Check sheet for the modelled part. Datum: model origin and axes. Units: mm. Face numbers are marked on the shaded views. Coordinates: 2 decimals unless noted, no trailing zeros. Order: outer loops, then holes, each group sorted by start corner. A loop starts at its lowest first (then second) coordinate and runs counter-clockwise, first axis right, second up. Notation, with made-up numbers: M 67.25,-1.5 L 104.25,-1.5 A25 ccw 104.25,18.5 Z; hole C 85.25,-40 d9. An arc over 180 degrees is marked long. Answer in a Markdown table with one row per item. Add a question column.
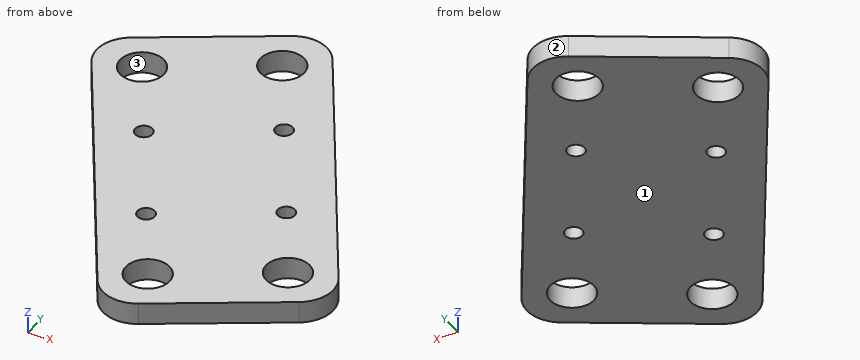
from build123d import *

# Parameters (mm, degrees)
SKETCH1_R           = 3.175
BOSS_EXTRUDE1_DEPTH = 3.175


with BuildPart() as part:
    # Sketch1 → Boss-Extrude1 (new body)
    with BuildSketch(Plane.XY):
        with BuildLine():
            Line((-86.435913995, -165.602360031), (-61.825632619, -205.632275727))
            ThreePointArc((-61.825632619, -205.632275727), (-58.676812327, -207.913058463), (-54.837503206, -207.299263221))
            Line((-54.837503206, -207.299263221), (-37.614442835, -196.710573375))
            ThreePointArc((-37.614442835, -196.710573375), (-35.333660099, -193.561753082), (-35.947455341, -189.722443962))
            Line((-35.947455341, -189.722443962), (-60.557736717, -149.692528266))
            ThreePointArc((-60.557736717, -149.692528266), (-63.706557009, -147.411745529), (-67.54586613, -148.025540772))
            Line((-67.54586613, -148.025540772), (-84.768926501, -158.614230618))
            ThreePointArc((-84.768926501, -158.614230618), (-87.049709237, -161.763050911), (-86.435913995, -165.602360031))
        make_face()
        with Locations((-80.361323188, -163.358535945)):
            Circle(SKETCH1_R, mode=Mode.SUBTRACT)
        with Locations((-65.302042044, -154.100131579)):
            Circle(SKETCH1_R, mode=Mode.SUBTRACT)
        with Locations((-42.022046148, -191.966268048)):
            Circle(SKETCH1_R, mode=Mode.SUBTRACT)
        with Locations((-57.081327292, -201.224672414)):
            Circle(SKETCH1_R, mode=Mode.SUBTRACT)
        with BuildLine():
            ThreePointArc((-62.635083896, -190.503539682), (-63.560924333, -188.997611568), (-65.066852447, -189.923452004))
            ThreePointArc((-65.066852447, -189.923452004), (-64.141012011, -191.429380119), (-62.635083896, -190.503539682))
        make_face(mode=Mode.SUBTRACT)
        with BuildLine():
            ThreePointArc((-50.007571303, -180.665047637), (-49.081730866, -182.170975752), (-47.575802752, -181.245135315))
            ThreePointArc((-47.575802752, -181.245135315), (-48.501643188, -179.739207201), (-50.007571303, -180.665047637))
        make_face(mode=Mode.SUBTRACT)
        with BuildLine():
            ThreePointArc((-56.834207119, -166.185854171), (-57.760047555, -164.679926057), (-59.26597567, -165.605766493))
            ThreePointArc((-59.26597567, -165.605766493), (-58.340135233, -167.111694608), (-56.834207119, -166.185854171))
        make_face(mode=Mode.SUBTRACT)
        with BuildLine():
            ThreePointArc((-74.325256814, -174.86417086), (-73.399416377, -176.370098974), (-71.893488263, -175.444258538))
            ThreePointArc((-71.893488263, -175.444258538), (-72.819328699, -173.938330423), (-74.325256814, -174.86417086))
        make_face(mode=Mode.SUBTRACT)
    extrude(amount=BOSS_EXTRUDE1_DEPTH)


solid = part.part
1. Go/stop test with flat-tipped pins: pin 1 Ø1.5 at (y, z) = (-156, 2) entering from +X; pin 2 Ø1 at (y, z) = (-200, 2.5) entering from +X. Record where each tip stops, or that it passes through.
2. Section check B-B on z = 0.5. State how many separate pieces and enclosed holes the cut face has, then the cut area to 3 significant figures.
3. Release check for a two-part mould opening along X. For the marked faces 1, 2 and 3 record: released by +X, released by -X, zero draft, split by the parting line, or undercut.
4. Section check D-D on y = -172. Enter the section's corners in (x, z) (3 decimals), then the cut area to 3 significant figures.
5. Scan lines: line 1 (Y direction, x = -64, z = 0.9); line 2 (X direction, y = -162, z = 1.95); line 3 (Y direction, x = -81, z = 2.3). Record each from-to range of solid material in increasing order.
6. Section check C-C on x = -82. Enter the section's corners in (y, z) (3 decimals).
7. Section check A-A on x = -44. Enter the section's corners in (y, z) (3 decimals).
Result sheet:
| question | item | result |
|---|---|---|
| 1 | pin 1 | x = -56.22 |
| 1 | pin 2 | x = -42.15 |
| 2 | separate pieces | 1 |
| 2 | enclosed holes | 8 |
| 2 | area | 1,570 mm^2 |
| 3 | face 1 | zero draft |
| 3 | face 2 | split by the parting line |
| 3 | face 3 | undercut |
| 4 | outline | M -82.503,0 L -46.843,0 L -46.843,3.175 L -82.503,3.175 Z |
| 4 | area | 113 mm^2 |
| 5 | line 1 | -202.1 to -191.45, -188.97 to -157, -151.2 to -147.35 |
| 5 | line 2 | -87.1 to -83.23, -77.49 to -52.99 |
| 5 | line 3 | -174.44 to -166.47, -160.25 to -156.3 |
| 6 | outline | M -172.818,0 L -166.078,0 L -166.078,3.175 L -172.818,3.175 Z; M -160.639,0 L -156.912,0 L -156.912,3.175 L -160.639,3.175 Z |
| 7 | outline | M -200.636,0 L -194.45,0 L -194.45,3.175 L -200.636,3.175 Z; M -189.483,0 L -176.625,0 L -176.625,3.175 L -189.483,3.175 Z |
